Input: part model. Units: mm. Frame: model coordinates. A direction names the side the tool comes from. Give positions to 0.01 mm unless a question says otherwise; leave off trailing zeros. Loops run counter-clockwise (first coordinate to the right, second up) from the corner with the lowest first, then second, coordinate; pieces in that order, holes last.
from build123d import *

# Parameters (mm, degrees)
PAD_DEPTH    = 2
SKETCH001_R  = 1.425
PAD001_DEPTH = 1
SKETCH002_R  = 1.425
PAD002_DEPTH = 5
SKETCH003_R  = 1.1
PAD003_DEPTH = 1.75
SKETCH004_R  = 1.375
PAD004_DEPTH = 5
SKETCH005_R  = 1.125
PAD005_DEPTH = 13.5
SKETCH006_W  = 92
SKETCH006_H  = 2.5
POCKET_DEPTH = 1
CHAMFER_SIZE = 0.5


with BuildPart() as part:
    # Sketch → Pad (new body)
    with BuildSketch(Plane.XZ):
        Polygon((0, 1.4), (12, 1.4), (12, 0.7), (24, 0.7), (24, 0), (68, 0), (68, 0.7), (80, 0.7), (80, 1.4), (92, 1.4), (92, 8.4), (11, 8.4), (11, 6.9), (0, 6.9), align=None)
    extrude(amount=PAD_DEPTH)

    # Sketch001 (on Face10 of Pad) → Pad001 (join)
    with BuildSketch(Plane(origin=(92, 0, 0), x_dir=(0, 0, 1), z_dir=(1, 0, 0))):
        with Locations((8.7, 0.6)):
            Circle(SKETCH001_R)
    extrude(amount=PAD001_DEPTH)

    # Sketch002 (on Face14 of Pad001) → Pad002 (join)
    with BuildSketch(Plane(origin=(92, 0, 0), x_dir=(0, 0, 1), z_dir=(1, 0, 0))):
        with Locations((8.7, 0.6)):
            Circle(SKETCH002_R)
    extrude(amount=-PAD002_DEPTH)

    # Sketch003 (on Face19 of Pad002) → Pad003 (join)
    with BuildSketch(Plane(origin=(93, 0, 0), x_dir=(0, 0, 1), z_dir=(1, 0, 0))):
        with Locations((8.7, 0.6)):
            Circle(SKETCH003_R)
    extrude(amount=PAD003_DEPTH)

    # Sketch004 (on Face18 of Pad003) → Pad004 (join)
    with BuildSketch(Plane(origin=(11, 0, 0), x_dir=(0, 0, -1), z_dir=(-1, 0, 0))):
        with Locations((-8.7, 0.6)):
            Circle(SKETCH004_R)
    extrude(amount=-PAD004_DEPTH)

    # Sketch005 (on Face23 of Pad004) → Pad005 (join)
    with BuildSketch(Plane(origin=(11, 0, 0), x_dir=(0, 0, -1), z_dir=(-1, 0, 0))):
        with Locations((-8.7, 0.6)):
            Circle(SKETCH005_R)
    extrude(amount=PAD005_DEPTH)

    # Sketch006 (on Face4 of Pad005) → Pocket (cut)
    with BuildSketch(Plane(origin=(0, 0, 0), x_dir=(1, 0, 0), z_dir=(0, 1, 0))):
        with Locations((46, -1.25)):
            Rectangle(SKETCH006_W, SKETCH006_H)
    extrude(amount=-POCKET_DEPTH, mode=Mode.SUBTRACT)

    # Chamfer
    chamfer_edges = [part.edges().sort_by_distance(p)[0] for p in [
        (46, -1, 0),
    ]]
    chamfer(chamfer_edges, length=CHAMFER_SIZE)


solid = part.part
(1) Ray query, probe 1 along X at (y, z) = (0.2, 9); probe 2 along X at (y, z) = (-0.6, 7); probe 3 along Z at (x, y) = (82.5, -0.45). Return the intervals inside material, ascending.
Values follow:
probe 1: x = -2.5 to 16, 87 to 94.75
probe 2: x = 11 to 92
probe 3: z = 2.5 to 8.4
(2) Cut plane C-C (x = 84). Return the cut outline in (y, z).
Values follow:
outline: (-2, 1.4) - (-1, 1.4) - (-1, 2.5) - (0, 2.5) - (0, 8.4) - (-2, 8.4) - close
(3) Reachability of faces 5 (the flat face through (45, -1, 1)), 6 (the cylindrical face through (93.863, -1.343, 7.889)), 7 (the cylindrical face through (4.34, -0.17, 7.66)) from +Z, -Z, +X, -X, +Y, -Y: full face, straight path, thin tool, end or side. Return the list, or none.
Values follow:
face 5: -Z, +X, -X, +Y
face 6: +X
face 7: -X
(4) Cut plane A-A (x = 45). Return the cut outline in (y, z).
Values follow:
outline: (-2, 0) - (-1.5, 0) - (-1, 0.5) - (-1, 2.5) - (0, 2.5) - (0, 8.4) - (-2, 8.4) - close
(5) Pin query (flat end, axial travel): pin 1 Ø3 at (x, z) = (15, 9) entering from -Y; pin 2 Ø1.1 at (x, y) = (5.5, -1.5) entering from -Z; pin 3 Ø3 at (x, z) = (35.5, 5.5) entering from +Y. Return the tip coordinate at first contact, or that it passes through.
Values follow:
pin 1: stops at y = -2
pin 2: stops at z = 1.4
pin 3: stops at y = 0
(6) Cut plane B-B (z = 5.5). Return the cut outline in (x, y), and give its area (3 significant figures).
Values follow:
outline: (0, -2) - (92, -2) - (92, 0) - (0, 0) - close
area: 184 mm2
(7) Mould query, pull axis X, two halves, no side actions, for faces 1 (the flat face through (11, -0.9, 7.45)), 2 (the flat face through (6, -1, 6.9)), 3 (the flat face through (92, -1, 5)), 4 (the flat face through (16, -1, 9)). Classes: +X half, -X half, draft (parallel to the pull), parting line (faces both ways), or undercut.
Values follow:
face 1: -X half
face 2: draft
face 3: +X half
face 4: undercut
